Autodesk Inventor part; units mm, degrees
ref_plane "YZ Plane" through (0, 0, 0) normal (1, 0, 0) x (0, 1, 0)
ref_plane "XZ Plane" through (0, 0, 0) normal (0, 1, 0) x (-1, 0, 0)
ref_plane "XY Plane" through (0, 0, 0) normal (0, 0, 1) x (1, 0, 0)
sketch "Sketch1" plane through (0, 0, 0) normal (0, 1, 0) x (-1, 0, 0)
  arc A0 (38.1, -38.2321) -> (-38.1, -38.2321) centre (0, 0) ccw
  line L0 (0, 0) -> (0, -72.7817) construction
  line L1 (-38.1, -38.2321) -> (-38.1, -69.85)
  line L2 (-38.1, -69.85) -> (0, -69.85)
  line L3 (0, -69.85) -> (38.1, -69.85)
  line L4 (38.1, -69.85) -> (38.1, -38.2321)
  dimension "d0" = 107.95
  dimension "d6" = 69.85
  dimension "d7" = 38.1
extrude "Extrusion1" add sketch "Sketch1" along normal blind 6.35
sketch "Sketch3" plane through (0, 0, 0) normal (0, -1, 0) x (1, 0, 0)
  arc A0 (38.1, -38.2321) -> (-38.1, -38.2321) centre (0, 0) ccw
  line L0 (38.1, -38.2321) -> (38.1, -69.85)
  line L1 (38.1, -69.85) -> (-38.1, -69.85)
  line L2 (-38.1, -69.85) -> (-38.1, -38.2321)
  arc A1 (38.1, -38.2321) -> (-38.1, -38.2321) centre (0, 0) ccw
  line L3 (38.1, -38.2321) -> (38.1, -69.85)
  line L4 (38.1, -38.2321) -> (38.1, -69.85)
  line L5 (38.1, -69.85) -> (-38.1, -69.85)
  line L6 (-38.1, -69.85) -> (-38.1, -38.2321)
  line L7 (-38.1, -69.85) -> (-38.1, -38.2321)
  arc A2 (44.45, -40.7836) -> (-44.45, -40.7836) centre (0, 0) ccw
  line L8 (44.45, -40.7836) -> (44.45, -76.2)
  line L9 (44.45, -76.2) -> (-44.45, -76.2)
  line L10 (-44.45, -76.2) -> (-44.45, -40.7836)
  dimension "d8" = 6.35
  dimension "d9" = 6.35
  dimension "d10" = 6.35
  dimension "d11" = 6.35
extrude "Extrusion4" add sketch "Sketch3" against normal blind 6.35
sketch "Sketch5" plane through (0, 6.35, 0) normal (0, 1, 0) x (1, 0, 0)
  circle A0 centre (0, 0) radius 12.7
  dimension "d24" = 25.4
extrude "Extrusion7" cut sketch "Sketch5" against normal through all
equation "\"d0\" = exteriorDiameter"
equation "\"exteriorDiameter\" = 107.95"
properties part number "baseSupportCover"
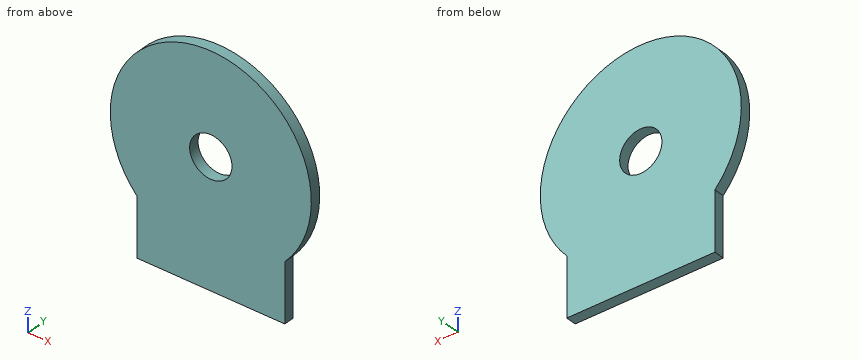
Check sheet for the modelled part. Datum: model origin and axes. Units: mm. Give positions to 0.01 mm unless a question says otherwise; leave off trailing zeros. Loops run counter-clockwise (first coordinate to the right, second up) from the corner with the lowest first, then second, coordinate; pieces in that order, holes last. Notation, with made-up numbers: M -33.75,38.5 L -1.75,38.5 A31 cw -1.75,71.5 Z; hole C 37,-1.5 d8. An arc over 180 degrees is marked long. Use a Markdown table: item, result. Add a question column.
Q1. Sectioned sample at A-A, the plane x = 0. Record the cut outline in (y, z) (3 decimals).
Q2. Go/stop test with flat-tipped pins: pin 1 (3 mm diameter, centred on y = 2, z = -60, fed in from -X); pin 2 (1.5 mm diameter, centred on y = 1.5, z = -38.5, fed in from -X). Record where each tip stops, or that it passes through.
Q3. Sectioned sample at D-D, the plane x = 34. Record the cut outline in (y, z), then the cut area to 3 significant figures.
Q4. Scan lines: line 1 along X through (y, z) = (4.5, 0) (3 decimals); line 2 along Z through (x, y) = (0, 3) (3 decimals); line 3 along Z through (x, y) = (5.5, 4). Record each from-to range of solid material in increasing order. Write a range as [from, to].
Q5. Sectioned sample at C-C, the plane z = 10.5. Record the cut outline in (x, y), then the cut area to 3 significant figures.
Q6. Sectioned sample at B-B, the plane y = 3. Record the cut outline in (x, z) (3 decimals).
Verdict:
| question | item | result |
|---|---|---|
| 1 | outline | M 0,-76.2 L 6.35,-76.2 L 6.35,-12.7 L 0,-12.7 Z; M 0,12.7 L 6.35,12.7 L 6.35,60.325 L 0,60.325 Z |
| 2 | pin 1 | x = -44.45 |
| 2 | pin 2 | x = -47.05 |
| 3 | outline | M 0,-76.2 L 6.35,-76.2 L 6.35,49.83 L 0,49.83 Z |
| 3 | area | 800 mm^2 |
| 4 | line 1 | [-60.325, -12.7], [12.7, 60.325] |
| 4 | line 2 | [-76.2, -12.7], [12.7, 60.325] |
| 4 | line 3 | [-76.2, -11.45], [11.45, 60.07] |
| 5 | outline | M -59.4,0 L -7.14,0 L -7.14,6.35 L -59.4,6.35 Z; M 7.14,0 L 59.4,0 L 59.4,6.35 L 7.14,6.35 Z |
| 5 | area | 664 mm^2 |
| 6 | outline | M -44.45,-76.2 L 44.45,-76.2 L 44.45,-40.784 A60.325 ccw long -44.45,-40.784 Z; hole C 0,0 d25.4 |
